```python
from build123d import *

# Parameters (mm, degrees)
SKETCH1_R           = 14.2875
SKETCH1_R_2         = 2.4892
BOSS_EXTRUDE1_DEPTH = 3.175


with BuildPart() as part:
    # Sketch1 → Boss-Extrude1 (new, symmetric)
    with BuildSketch(Plane.XY):
        with BuildLine():
            Line((-25.711392616, 16.628788534), (-19.959064153, -5.248062916))
            ThreePointArc((-19.959064153, -5.248062916), (-7.46638511, -19.239529611), (11.194044807, -17.337813216))
            Line((11.194044807, -17.337813216), (30.197779716, -5.06817705))
            ThreePointArc((30.197779716, -5.06817705), (31.796268643, -3.513762679), (32.671001067, -1.462857007))
            Line((32.671001067, -1.462857007), (44.467361552, 55.261864273))
            ThreePointArc((44.467361552, 55.261864273), (43.898602792, 59.119668038), (40.971040985, 61.695618015))
            Line((40.971040985, 61.695618015), (11.371764661, 73.182364338))
            ThreePointArc((11.371764661, 73.182364338), (7.472947104, 73.255563185), (4.450757502, 70.791317575))
            Line((4.450757502, 70.791317575), (-25.105168777, 20.958644089))
            ThreePointArc((-25.105168777, 20.958644089), (-25.842883045, 18.854565063), (-25.711392616, 16.628788534))
        make_face()
        Circle(SKETCH1_R, mode=Mode.SUBTRACT)
        with Locations((13.784095588, 35.519131589)):
            Circle(SKETCH1_R, mode=Mode.SUBTRACT)
        with Locations((-20.233397162, 18.069179956)):
            Circle(SKETCH1_R_2, mode=Mode.SUBTRACT)
        with Locations((27.125444956, -0.309614161)):
            Circle(SKETCH1_R_2, mode=Mode.SUBTRACT)
        with Locations((38.921805441, 56.415107119)):
            Circle(SKETCH1_R_2, mode=Mode.SUBTRACT)
        with Locations((9.322529117, 67.901853442)):
            Circle(SKETCH1_R_2, mode=Mode.SUBTRACT)
    extrude(amount=BOSS_EXTRUDE1_DEPTH, both=True)


solid = part.part
```
For this review, take the finished solid that the model builds, in its own axes (mm). Round coordinates to 2 decimals unless told otherwise and drop trailing zeros. Order: outer loops, then holes, each group sorted by start corner. A loop starts at its lowest first (then second) coordinate and runs counter-clockwise, first axis right, second up. Notation, with made-up numbers: (34, -20.75) -> (80, -20.75) arc R35 cw to (80, 14.25) -> close; hole circle Ø2 at (24, 51.25). An arc over 180 degrees is marked (long way). Use a Markdown table: item, result.
Item 1: Take a section at C-C (z = 1). State the section outline as (x, y) points (1 decimal), plus the area to 3 significant figures.
Resolved:
| item | result |
|---|---|
| outline | (-25.7, 16.6) -> (-20, -5.2) arc R20.6 ccw to (11.2, -17.3) -> (30.2, -5.1) arc R5.7 ccw to (32.7, -1.5) -> (44.5, 55.3) arc R5.7 ccw to (41, 61.7) -> (11.4, 73.2) arc R5.7 ccw to (4.5, 70.8) -> (-25.1, 21) arc R5.7 ccw to start; hole circle Ø5 at (-20.2, 18.1); hole circle Ø28.6 at (0, 0); hole circle Ø28.6 at (13.8, 35.5); hole circle Ø5 at (9.3, 67.9); hole circle Ø5 at (27.1, -0.3); hole circle Ø5 at (38.9, 56.4) |
| area | 3,140 mm² |
Item 2: For pin 1 (17 mm diameter, centred on x = 13.78, y = 35.52, fed in from +Z); pin 2 (1 mm diameter, centred on x = 32, z = 0, fed in from +Y); pin 3 (3 mm diameter, centred on x = 17, z = -1, fed in from +Y); pin 4 (3 mm diameter, centred on y = 63, z = -0.5, fed in from +X), all flat-tipped, find the tip position at first contact; note any pin that passes through.
Resolved:
| item | result |
|---|---|
| pin 1 | passes through |
| pin 2 | stops at y = 65.37 |
| pin 3 | stops at y = 71.58 |
| pin 4 | stops at x = 41.42 |
Item 3: Take a section at D-D (y = 51.5). State the section outline as (x, z) points (3 decimals).
Resolved:
| item | result |
|---|---|
| outline | (-6.991, -3.175) -> (43.685, -3.175) -> (43.685, 3.175) -> (-6.991, 3.175) -> close |
Item 4: Take a section at B-B (y = 30). State the section outline as (x, z) points (3 decimals).
Resolved:
| item | result |
|---|---|
| outline | (-19.743, -3.175) -> (0.606, -3.175) -> (0.606, 3.175) -> (-19.743, 3.175) -> close; (26.963, -3.175) -> (39.214, -3.175) -> (39.214, 3.175) -> (26.963, 3.175) -> close |
Item 5: Take a section at A-A (x = 19.5). State the section outline as (y, z) points (3 decimals).
Resolved:
| item | result |
|---|---|
| outline | (-11.975, -3.175) -> (22.425, -3.175) -> (22.425, 3.175) -> (-11.975, 3.175) -> close; (48.613, -3.175) -> (70.028, -3.175) -> (70.028, 3.175) -> (48.613, 3.175) -> close |
Item 6: For line 1 along Y through (x, z) = (8.5, 3); line 2 along X through (y, z) = (-1, 1.25); line 3 along Y through (x, z) = (-11.5, -1.5), list the stretches that pass through material, from the lowest coordinate up. Write a range as [from, to].
Resolved:
| item | result |
|---|---|
| line 1 | y = [-18.81, -11.48], [11.48, 22.24], [48.79, 65.55], [70.25, 73.51] |
| line 2 | x = [-21.08, -14.25], [14.25, 24.73], [29.52, 32.77] |
| line 3 | y = [-17.14, -8.48], [8.48, 43.9] |
Item 7: Draft analysis for pull direction Y (two halves, no side actions). For faces 1 (the cylindrical face through (-7.72, -19.14, 0.04)), 2 (the cylindrical face through (29.5, 0.44, -0.04)), 3 (the cylindrical face through (-25.838, 18.886, 0.044)), state which applies: +Y half, -Y half, draft (parallel to the pull), parting line (faces both ways), or undercut.
Resolved:
| item | result |
|---|---|
| face 1 | -Y half |
| face 2 | undercut |
| face 3 | parting line |
